from build123d import *

# Parameters (mm, degrees)
BOX001_W        = 74
BOX001_H        = 71
BOX001_DEPTH    = 1
SKETCH016_W     = 50
SKETCH016_H     = 50
POCKET009_DEPTH = 1.001
FILLET001_R     = 19


with BuildPart() as part:
    # Box001 → Box001 (new body)
    with BuildSketch(Plane(origin=(2, 0, 1), x_dir=(1, 0, 0), z_dir=(0, 0, 1))):
        with Locations((37, 35.5)):
            Rectangle(BOX001_W, BOX001_H)
    extrude(amount=BOX001_DEPTH)


with BuildPart() as part_1:
    # BaseFeature001 placement: moved
    add(part.part.moved(Location((-2, 0, -1))))

    # Sketch016 (on Face6 of BaseFeature001) → Pocket009 (cut, through all)
    with BuildSketch(Plane.XY.offset(1)):
        with Locations((37, 46)):
            Rectangle(SKETCH016_W, SKETCH016_H)
    extrude(amount=-POCKET009_DEPTH, mode=Mode.SUBTRACT)

    # Fillet001
    fillet001_edges = [part_1.edges().sort_by_distance(p)[0] for p in [
        (12, 21, 0.5),
        (62, 21, 0.5),
    ]]
    fillet(fillet001_edges, radius=FILLET001_R)


with BuildPart() as part_2:
    # Body001 placement: moved
    add(part_1.part.moved(Location((0, -89, 0))))


solid = part_2.part
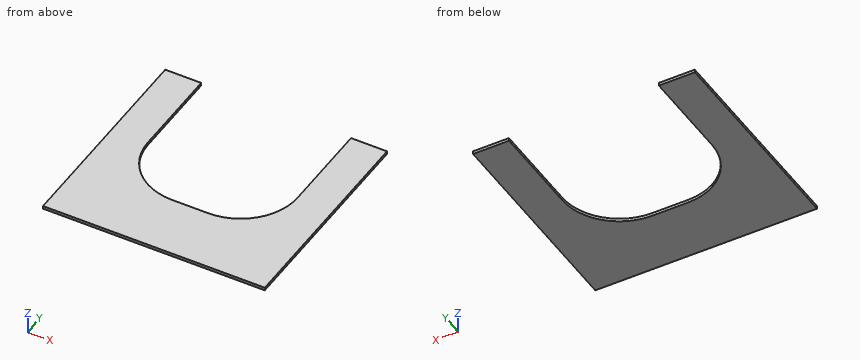
For this review, take the finished solid that the model builds, in its own axes (mm). Give positions to 0.01 mm unless a question says otherwise; leave off trailing zeros. Order: outer loops, then holes, each group sorted by start corner. A loop starts at its lowest first (then second) coordinate and runs counter-clockwise, first axis right, second up. Notation, with made-up numbers: (18, 75) - (60, 75) arc R33 ccw to (60, 114) - close; hole circle Ø8 at (20, 58). An arc over 180 degrees is marked (long way). Answer as a JSON object with one key per item and string values. Group by question number.
Item 1: Take a section at B-B on z = 0.35. Give the boundary of the cut face in (x, y).
Item 2: Take a section at A-A on y = -28. Give the boundary of the cut face in (x, z).
Item 3: Take a section at C-C on x = 40. Give the boundary of the cut face in (y, z).
Item 4: Take a section at D-D on y = -56. Give the boundary of the cut face in (x, z), and give its area (3 significant figures).
Item 5: Wall thickness on line 1 along X through (y, z) = (-45, 0.35); line 2 along X through (y, z) = (-53.5, 0.4); line 3 along Y through (x, z) = (40.5, 0.8): over which ranges is each line inside the solid? List them lowest first.
Item 6: Clearance check with a flat-ended pin moving along its axis: pin 1 Ø0.5 at (x, z) = (36.5, 0.5) entering from +Y. State where the tip first meets the part, or that it passes through.
Reported:
{
 "1": {"outline": "(0, -89) - (74, -89) - (74, -18) - (62, -18) - (62, -49) arc R19 cw to (43, -68) - (31, -68) arc R19 cw to (12, -49) - (12, -18) - (0, -18) - close"},
 "2": {"outline": "(0, 0) - (12, 0) - (12, 1) - (0, 1) - close; (62, 0) - (74, 0) - (74, 1) - (62, 1) - close"},
 "3": {"outline": "(-89, 0) - (-68, 0) - (-68, 1) - (-89, 1) - close"},
 "4": {"outline": "(0, 0) - (13.34, 0) - (13.34, 1) - (0, 1) - close; (60.66, 0) - (74, 0) - (74, 1) - (60.66, 1) - close", "area": "26.7 mm^2"},
 "5": {"line 1": "0 to 12, 62 to 74", "line 2": "0 to 12.54, 61.46 to 74", "line 3": "-89 to -68"},
 "6": {"pin 1": "y = -68"}
}
